```python
from build123d import *

# Parameters (mm, degrees)
F0_R     = 3.5
F0_R_2   = 1.575
F1_DEPTH = 2.2
F2_DEPTH = 4


# Not quite as in the source:
# - a fillet or chamfer that OpenCascade refuses, or shapes differently, is made with other operations: its cross-section is extruded or revolved along the edge and cut away or added


with BuildPart() as f1:
    # F0 (on Front) → F1 (new body)
    with BuildSketch(Plane.XZ):
        Circle(F0_R)
        Circle(F0_R_2, mode=Mode.SUBTRACT)
        Circle(F0_R_2)
    extrude(amount=F1_DEPTH)

    # F0 (on Front) → F2 (cut)
    with BuildSketch(Plane.XZ):
        Circle(F0_R_2)
    extrude(amount=F2_DEPTH, mode=Mode.SUBTRACT)

    # F3: chamfer of 2 on 1 edges, made by hand

    # F3_s1 → F3_t2 (revolve, cut)
    with BuildSketch(Plane.XY):
        Polygon((3.575, -2.2), (1.575, -0.2), (1.575, -2.2), align=None)
    revolve(axis=Axis((0, -2.2, 0), (0, 1, 0)), mode=Mode.SUBTRACT)


solid = f1.part
```
Check sheet for the modelled part. Datum: model origin and axes. Units: mm. Coordinates: 2 decimals unless noted, no trailing zeros. Write each loop counter-clockwise with the first axis right and the second up, starting at its lowest first coordinate (ties: lowest second). Pieces come first, ordered by that corner, then holes. Notation, with made-up numbers: (39, 78.5) - (61, 78.5) arc R33 cw to (61, 116.5) - close; hole circle Ø4 at (84, 3.5). An arc over 180 degrees is marked (long way). One line per question, with ' | ' between items.
Item 1: Sectioned sample at D-D on y = -0.65. Record the boundary of the cut face in (x, z) (3 decimals).
Determined:
outline: circle Ø7 at (0, 0); hole circle Ø4.05 at (0, 0)
Item 2: Sectioned sample at B-B on x = 0. Record the boundary of the cut face in (y, z) (3 decimals).
Determined:
outline: (-2.125, -3.5) - (0, -3.5) - (0, -1.575) - (-0.2, -1.575) - close; (-2.125, 3.5) - (-0.2, 1.575) - (0, 1.575) - (0, 3.5) - close
Item 3: Sectioned sample at A-A on z = 0. Record the boundary of the cut face in (x, y) (3 decimals).
Determined:
outline: (-3.5, -2.125) - (-1.575, -0.2) - (-1.575, 0) - (-3.5, 0) - close; (1.575, -0.2) - (3.5, -2.125) - (3.5, 0) - (1.575, 0) - close
Item 4: Sectioned sample at C-C on y = -1.45. Record the boundary of the cut face in (x, z) (3 decimals).
Determined:
outline: circle Ø7 at (0, 0); hole circle Ø5.65 at (0, 0)
Item 5: Thickness scan on line 1 (X direction, y = -0.05, z = 0) (3 decimals); line 2 (X direction, y = -0.7, z = -0.5). Record the ranges inside material, lowest first. Write a range as [from, to].
Determined:
line 1: x = [-3.5, -1.575], [1.575, 3.5] | line 2: x = [-3.46, -2.01], [2.01, 3.46]
